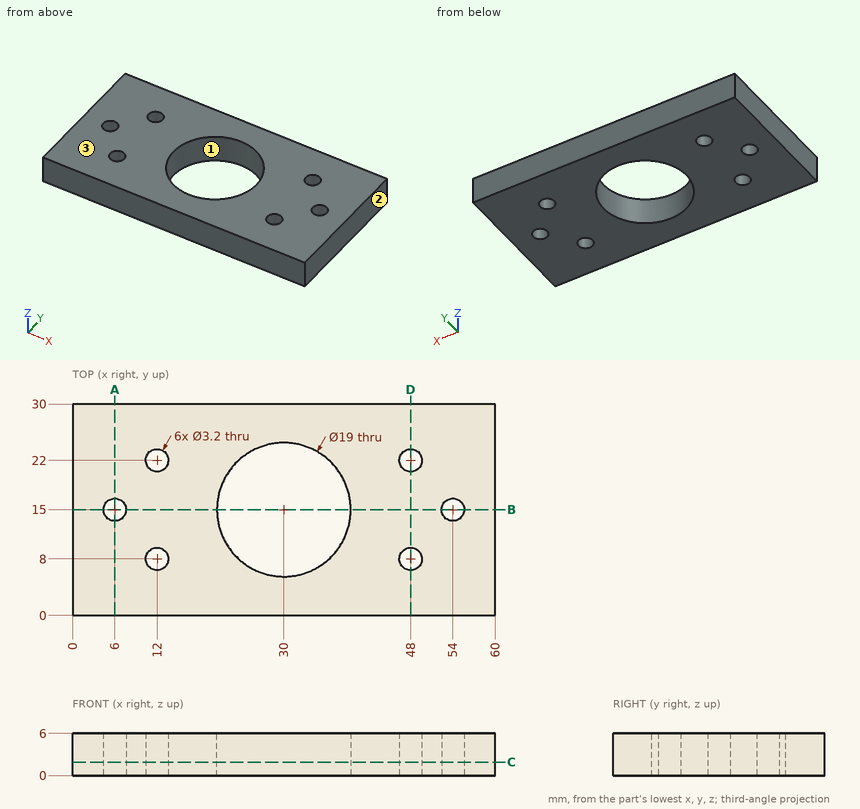
Geometry: see drawing. Coordinates: mm, zero at the bounding-box minimum. Give positions to 0.01 mm unless a question says otherwise; leave off trailing zeros. Order: outer loops, then holes, each group sorted by start corner. A loop starts at its lowest first (then second) coordinate and runs counter-clockwise, first axis right, second up. Notation, with made-up numbers: M 54,40 L 86,40 A14 cw 86,61 Z; hole C -25.5,44.5 d8. An arc over 180 degrees is marked long. Answer as CSV lines item,"result". Start each with the question number.
1) Line query: line 1 (Y direction, x = 48, z = 3.8); line 2 (X direction, y = 22, z = 3.5); line 3 (Y direction, x = 6, z = 4.5). Output: solid intervals per line, ascending. Write a range as from..to.
2) Mould query, pull axis X, two halves, no side actions, for the marked faces 1, 2 and 3. Classes: +X half, -X half, draft (parallel to the pull), parting line (faces both ways), or undercut.
3) Cut plane B-B (y = 15). Output: boundary loops of the cut face in (x, z).
4) Cut plane A-A (x = 6). Output: boundary loops of the cut face in (y, z), then the cut area to 3 significant figures.
5) Cut plane C-C (z = 1.9). Output: boundary loops of the cut face in (x, y).
6) Cut plane D-D (x = 48). Output: boundary loops of the cut face in (y, z), then the cut area to 3 significant figures.
Findings below:
1,line 1,"y = 0..6.4, 9.6..20.4, 23.6..30"
1,line 2,"x = 0..10.4, 13.6..23.58, 36.42..46.4, 49.6..60"
1,line 3,"y = 0..13.4, 16.6..30"
2,face 1,"undercut"
2,face 2,"+X half"
2,face 3,"draft"
3,outline,"M 0,0 L 4.4,0 L 4.4,6 L 0,6 Z; M 7.6,0 L 20.5,0 L 20.5,6 L 7.6,6 Z; M 39.5,0 L 52.4,0 L 52.4,6 L 39.5,6 Z; M 55.6,0 L 60,0 L 60,6 L 55.6,6 Z"
4,outline,"M 0,0 L 13.4,0 L 13.4,6 L 0,6 Z; M 16.6,0 L 30,0 L 30,6 L 16.6,6 Z"
4,area,"161 mm²"
5,outline,"M 0,0 L 60,0 L 60,30 L 0,30 Z; hole C 6,15 d3.2; hole C 12,8 d3.2; hole C 12,22 d3.2; hole C 30,15 d19; hole C 48,8 d3.2; hole C 48,22 d3.2; hole C 54,15 d3.2"
6,outline,"M 0,0 L 6.4,0 L 6.4,6 L 0,6 Z; M 9.6,0 L 20.4,0 L 20.4,6 L 9.6,6 Z; M 23.6,0 L 30,0 L 30,6 L 23.6,6 Z"
6,area,"142 mm²"
